Build history of the part. All positions in model axes, mm. Face numbers are marked on the shaded views. A direction names the side the tool comes from. Give positions to 0.01 mm unless a question says otherwise; leave off trailing zeros. Write each loop counter-clockwise with the first axis right and the second up, starting at its lowest first coordinate (ties: lowest second). Pieces come first, ordered by that corner, then holes. Notation, with made-up numbers: M 66,-34.5 L 112,-34.5 A21 ccw 112,-13.5 Z; hole C -28.5,-26.75 d5. An arc over 180 degrees is marked long. Return JSON: item names as keys, results as strings. Group by question number.
Q1. Band-saw the part on A-A, the plane y = 8.75. Count the separate pieces of the cut face and the enclosed holes in it, then the cut area to 3 significant figures.
Q2. Pull direction Z, two halves, no side cores. Call the marked faces 1 and 2: +Z half, -Z half, draft (parallel to the pull), parting line (faces both ways), or undercut.
Q3. Wall check: probe 1 along X at (y, z) = (0.75, 21.5); probe 2 along Z at (x, y) = (17, 1); probe 3 along Z at (x, y) = (-1, 2). Give the ranges that are in metal, low to high.
Q4. Band-saw the part on B-B, the plane z = -17. Give the cut face in (x, y).
Q5. Flat gauge pins, fed straight in: pin 1 Ø0.8 at (x, z) = (8, 10.5) entering from +Y; pin 2 Ø0.6 at (x, y) = (-14.5, 4) entering from -Z; pin 3 Ø1.7 at (x, z) = (8.5, -6.5) entering from +Y. Where does each tip first touch, or does it go through?
Q6. Tool access for the marked faces 3 and 4: list every direction of +Z, -Z, +X, -X, +Y, -Y with a clear straight run to the whole face (end or side of a thin tool).
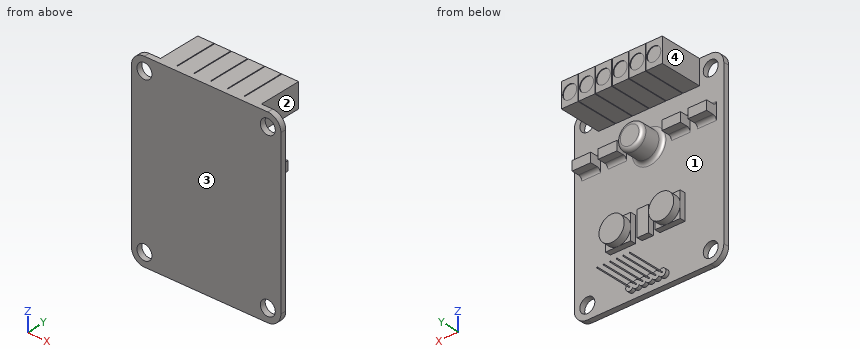
from build123d import *

# Parameters (mm, degrees)
SKETCH1_W           = 40
SKETCH1_H           = 50
BOSS_EXTRUDE1_DEPTH = 1.5
FILLET1_R           = 3.5
SKETCH2_R           = 2
CUT_EXTRUDE1_DEPTH  = 1.5
SKETCH3_W           = 27
SKETCH3_H           = 6.5
BOSS_EXTRUDE2_DEPTH = 11.5
SKETCH4_R           = 1.875
CUT_EXTRUDE2_DEPTH  = 0.2
SKETCH5_W           = 0.2
SKETCH5_H           = 6.5
CUT_EXTRUDE3_DEPTH  = 11.5
SKETCH6_R           = 3.5
BOSS_EXTRUDE3_DEPTH = 6
FILLET2_R           = 1
SKETCH7_W           = 5
SKETCH7_H           = 2.5
BOSS_EXTRUDE4_DEPTH = 3
FILLET3_R           = 1
BOSS_EXTRUDE5_DEPTH = 1
SKETCH9_R           = 0.125
BOSS_EXTRUDE6_DEPTH = 10
SKETCH10_W          = 6.75
SKETCH10_H          = 6.75
SKETCH10_W_2        = 3
BOSS_EXTRUDE7_DEPTH = 1.5
SKETCH11_R          = 3.375
BOSS_EXTRUDE8_DEPTH = 2


with BuildPart() as part:
    # Sketch1 → Boss-Extrude1 (new body)
    with BuildSketch(Plane(origin=(0, 0, 0), x_dir=(1, 0, 0), z_dir=(0, 1, 0))):
        Rectangle(SKETCH1_W, SKETCH1_H)
    extrude(amount=BOSS_EXTRUDE1_DEPTH)

    # Fillet1
    fillet1_edges = [part.edges().sort_by_distance(p)[0] for p in [
        (20, 0.75, 25),
        (-20, 0.75, 25),
        (-20, 0.75, -25),
        (20, 0.75, -25),
    ]]
    fillet(fillet1_edges, radius=FILLET1_R)

    # Sketch2 → Cut-Extrude1 (cut)
    with BuildSketch(Plane(origin=(0, 1.5, 0), x_dir=(1, 0, 0), z_dir=(0, 1, 0))):
        with Locations(Location((-16.5, 21.5, 0), (0, 0, 270))):
            Circle(SKETCH2_R)
        with Locations(Location((16.5, 21.5, 0), (0, 0, 270))):
            Circle(SKETCH2_R)
        with Locations(Location((-16.5, -21.5, 0), (0, 0, 270))):
            Circle(SKETCH2_R)
        with Locations(Location((16.5, -21.5, 0), (0, 0, 270))):
            Circle(SKETCH2_R)
    extrude(amount=-CUT_EXTRUDE1_DEPTH, mode=Mode.SUBTRACT)

    # Sketch3 → Boss-Extrude2 (add)
    with BuildSketch(Plane(origin=(0, 1.5, 0), x_dir=(1, 0, 0), z_dir=(0, 1, 0))):
        with Locations((0, -21.75)):
            Rectangle(SKETCH3_W, SKETCH3_H)
    extrude(amount=BOSS_EXTRUDE2_DEPTH)

    # Sketch4 → Cut-Extrude2 (cut)
    with BuildSketch(Plane(origin=(0, 13, 0), x_dir=(1, 0, 0), z_dir=(0, 1, 0))):
        with Locations(Location((-11.228178801, -21.670447507, 0), (0, 0, 270))):
            Circle(SKETCH4_R)
        with Locations(Location((-6.728178801, -21.670447507, 0), (0, 0, 270))):
            Circle(SKETCH4_R)
        with Locations(Location((-2.228178801, -21.670447507, 0), (0, 0, 270))):
            Circle(SKETCH4_R)
        with Locations(Location((2.271821199, -21.670447507, 0), (0, 0, 270))):
            Circle(SKETCH4_R)
        with Locations(Location((6.771821199, -21.670447507, 0), (0, 0, 270))):
            Circle(SKETCH4_R)
        with Locations(Location((11.271821199, -21.670447507, 0), (0, 0, 270))):
            Circle(SKETCH4_R)
    extrude(amount=-CUT_EXTRUDE2_DEPTH, mode=Mode.SUBTRACT)

    # Sketch5 → Cut-Extrude3 (cut)
    with BuildSketch(Plane(origin=(0, 13, 0), x_dir=(1, 0, 0), z_dir=(0, 1, 0))):
        with Locations((-9.045617119, -21.75)):
            Rectangle(SKETCH5_W, SKETCH5_H)
        with Locations((-4.545617119, -21.75)):
            Rectangle(SKETCH5_W, SKETCH5_H)
        with Locations((-0.045617119, -21.75)):
            Rectangle(SKETCH5_W, SKETCH5_H)
        with Locations((4.454382881, -21.75)):
            Rectangle(SKETCH5_W, SKETCH5_H)
        with Locations((8.954382881, -21.75)):
            Rectangle(SKETCH5_W, SKETCH5_H)
    extrude(amount=-CUT_EXTRUDE3_DEPTH, mode=Mode.SUBTRACT)

    # Sketch6 → Boss-Extrude3 (add)
    with BuildSketch(Plane(origin=(0, 1.5, 0), x_dir=(1, 0, 0), z_dir=(0, 1, 0))):
        with Locations(Location((0, -9.436720639, 0), (0, 0, 270))):
            Circle(SKETCH6_R)
    extrude(amount=BOSS_EXTRUDE3_DEPTH)

    # Fillet2
    fillet2_edges = [part.edges().sort_by_distance(p)[0] for p in [
        (0, 1.5, 5.936720639),
        (0, 7.5, 5.936720639),
    ]]
    fillet(fillet2_edges, radius=FILLET2_R)

    # Sketch7 → Boss-Extrude4 (add)
    with BuildSketch(Plane(origin=(0, 1.5, 0), x_dir=(1, 0, 0), z_dir=(0, 1, 0))):
        with Locations((-8.5, -10.75)):
            Rectangle(SKETCH7_W, SKETCH7_H)
        with Locations((-15.5, -10.75)):
            Rectangle(SKETCH7_W, SKETCH7_H)
        with Locations((8.5, -10.75)):
            Rectangle(SKETCH7_W, SKETCH7_H)
        with Locations((15.5, -10.75)):
            Rectangle(SKETCH7_W, SKETCH7_H)
    extrude(amount=BOSS_EXTRUDE4_DEPTH)

    # Fillet3
    fillet3_edges = [part.edges().sort_by_distance(p)[0] for p in [
        (-8.5, 1.5, 9.5),
        (-8.5, 1.5, 12),
        (-15.5, 1.5, 9.5),
        (-15.5, 1.5, 12),
        (8.5, 1.5, 12),
        (8.5, 1.5, 9.5),
        (15.5, 1.5, 12),
        (15.5, 1.5, 9.5),
    ]]
    fillet(fillet3_edges, radius=FILLET3_R)

    # Sketch8 → Boss-Extrude5 (add)
    with BuildSketch(Plane(origin=(0, 1.5, 0), x_dir=(1, 0, 0), z_dir=(0, 1, 0))):
        with BuildLine():
            ThreePointArc((-3.5, 22.984122918), (-5.375, 22.5), (-3.5, 22.015877082))
            ThreePointArc((-3.5, 22.015877082), (-2.625, 21.5), (-1.75, 22.015877082))
            ThreePointArc((-1.75, 22.015877082), (-0.875, 21.5), (0, 22.015877082))
            ThreePointArc((0, 22.015877082), (0.875, 21.5), (1.75, 22.015877082))
            ThreePointArc((1.75, 22.015877082), (2.625, 21.5), (3.5, 22.015877082))
            ThreePointArc((3.5, 22.015877082), (5.375, 22.5), (3.5, 22.984122918))
            ThreePointArc((3.5, 22.984122918), (2.625, 23.5), (1.75, 22.984122918))
            ThreePointArc((1.75, 22.984122918), (0.875, 23.5), (0, 22.984122918))
            ThreePointArc((0, 22.984122918), (-0.875, 23.5), (-1.75, 22.984122918))
            ThreePointArc((-1.75, 22.984122918), (-2.625, 23.5), (-3.5, 22.984122918))
        make_face()
    extrude(amount=BOSS_EXTRUDE5_DEPTH)

    # Sketch9 → Boss-Extrude6 (add)
    with BuildSketch(Plane(origin=(0, 2.5, 0), x_dir=(1, 0, 0), z_dir=(0, 1, 0))):
        with Locations(Location((-4.375, 22.5, 0), (0, 0, 270))):
            Circle(SKETCH9_R)
        with Locations(Location((-2.625, 22.5, 0), (0, 0, 270))):
            Circle(SKETCH9_R)
        with Locations(Location((-0.875, 22.5, 0), (0, 0, 270))):
            Circle(SKETCH9_R)
        with Locations(Location((0.875, 22.5, 0), (0, 0, 270))):
            Circle(SKETCH9_R)
        with Locations(Location((2.625, 22.5, 0), (0, 0, 270))):
            Circle(SKETCH9_R)
        with Locations(Location((4.375, 22.5, 0), (0, 0, 270))):
            Circle(SKETCH9_R)
    extrude(amount=BOSS_EXTRUDE6_DEPTH)

    # Sketch10 → Boss-Extrude7 (add)
    with BuildSketch(Plane(origin=(0, 1.5, 0), x_dir=(1, 0, 0), z_dir=(0, 1, 0))):
        with Locations((6.987498071, 8.697159078)):
            Rectangle(SKETCH10_W, SKETCH10_H)
        with Locations((0.362498071, 8.697159078)):
            Rectangle(SKETCH10_W_2, SKETCH10_H)
        with Locations((-6.262501929, 8.697159078)):
            Rectangle(SKETCH10_W, SKETCH10_H)
    extrude(amount=BOSS_EXTRUDE7_DEPTH)

    # Sketch11 → Boss-Extrude8 (add)
    with BuildSketch(Plane(origin=(0, 3, 0), x_dir=(1, 0, 0), z_dir=(0, 1, 0))):
        with Locations(Location((-6.262501929, 8.697159078, 0), (0, 0, 270))):
            Circle(SKETCH11_R)
        with Locations(Location((6.987498071, 8.697159078, 0), (0, 0, 270))):
            Circle(SKETCH11_R)
    extrude(amount=BOSS_EXTRUDE8_DEPTH)


solid = part.part
From the geometry:
{
 "1": {"separate pieces": "12", "enclosed holes": "0", "area": "169 mm^2"},
 "2": {"face 1": "undercut", "face 2": "draft"},
 "3": {"probe 1": "x = -20 to -18.5, -14.5 to 14.5, 18.5 to 20", "probe 2": "z = -24.96 to -23.44, -19.56 to 19.56, 23.44 to 24.96", "probe 3": "z = -23.49 to -21.51, -12.07 to -5.32, 5.94 to 12.93, 18.5 to 25"},
 "4": {"outline": "M -20,0 L 20,0 L 20,1.5 L -20,1.5 Z"},
 "5": {"pin 1": "stops at y = 4.5", "pin 2": "stops at z = 9.5", "pin 3": "stops at y = 5"},
 "6": {"face 3": "+Z, -Z, +X, -X, -Y", "face 4": "+Z, -X, +Y"}
}
